CAD build for the part. Positions are in the model's coordinates, mm. A direction names the side the tool comes from. Coordinates: 2 decimals unless noted, no trailing zeros. Order: outer loops, then holes, each group sorted by start corner. A loop starts at its lowest first (then second) coordinate and runs counter-clockwise, first axis right, second up. Notation, with made-up numbers: M 80.5,-39.75 L 131.5,-39.75 A14 cw 131.5,-33.75 Z; hole C 43,62.5 d7. An arc over 180 degrees is marked long. One line per item, written item: value.
from build123d import *

# Parameters (mm, degrees)
F1_DEPTH = 40
F3_DEPTH = 360
F3_TAPER = -3
F4_SIZE  = 10


with BuildPart() as f1:
    # F0 (on Top) → F1 (new body)
    with BuildSketch(Plane.XY):
        with BuildLine():
            Line((348.3026485145, 356.2960825861), (-11.6973514855, 356.2960825861))
            ThreePointArc((-11.6973514855, 356.2960825861), (-25.8394871092, 350.4382182098), (-31.6973514855, 336.2960825861))
            Line((-31.6973514855, 336.2960825861), (-31.6973514855, -23.7039174139))
            ThreePointArc((-31.6973514855, -23.7039174139), (-25.8394871092, -37.8460530377), (-11.6973514855, -43.7039174139))
            Line((-11.6973514855, -43.7039174139), (348.3026485145, -43.7039174139))
            ThreePointArc((348.3026485145, -43.7039174139), (362.4447841382, -37.8460530377), (368.3026485145, -23.7039174139))
            Line((368.3026485145, -23.7039174139), (368.3026485145, 336.2960825861))
            ThreePointArc((368.3026485145, 336.2960825861), (362.4447841382, 350.4382182098), (348.3026485145, 356.2960825861))
        make_face()
    extrude(amount=F1_DEPTH)

    # F2 (on face) → F3 (join)
    with BuildSketch(Plane(origin=(0, 0, 0), x_dir=(1, 0, 0), z_dir=(0, 0, -1))):
        with BuildLine():
            Line((40.8026485145, 3.7039174139), (15.8026485145, 3.7039174139))
            ThreePointArc((15.8026485145, 3.7039174139), (10.4993476556, 1.5072182728), (8.3026485145, -3.7960825861))
            Line((8.3026485145, -3.7960825861), (8.3026485145, -28.7960825861))
            ThreePointArc((8.3026485145, -28.7960825861), (10.4993476556, -34.0993834449), (15.8026485145, -36.2960825861))
            Line((15.8026485145, -36.2960825861), (40.8026485145, -36.2960825861))
            ThreePointArc((40.8026485145, -36.2960825861), (46.1059493734, -34.0993834449), (48.3026485145, -28.7960825861))
            Line((48.3026485145, -28.7960825861), (48.3026485145, -3.7960825861))
            ThreePointArc((48.3026485145, -3.7960825861), (46.1059493734, 1.5072182728), (40.8026485145, 3.7039174139))
        make_face()
        with BuildLine():
            ThreePointArc((288.3026485145, -28.7960825861), (290.4993476556, -34.0993834449), (295.8026485145, -36.2960825861))
            Line((295.8026485145, -36.2960825861), (320.8026485145, -36.2960825861))
            ThreePointArc((320.8026485145, -36.2960825861), (326.1059493734, -34.0993834449), (328.3026485145, -28.7960825861))
            Line((328.3026485145, -28.7960825861), (328.3026485145, -3.7960825861))
            ThreePointArc((328.3026485145, -3.7960825861), (326.1059493734, 1.5072182728), (320.8026485145, 3.7039174139))
            Line((320.8026485145, 3.7039174139), (295.8026485145, 3.7039174139))
            ThreePointArc((295.8026485145, 3.7039174139), (290.4993476556, 1.5072182728), (288.3026485145, -3.7960825861))
            Line((288.3026485145, -3.7960825861), (288.3026485145, -28.7960825861))
        make_face()
        with BuildLine():
            ThreePointArc((288.3026485145, -308.7960825861), (290.4993476556, -314.0993834449), (295.8026485145, -316.2960825861))
            Line((295.8026485145, -316.2960825861), (320.8026485145, -316.2960825861))
            ThreePointArc((320.8026485145, -316.2960825861), (326.1059493734, -314.0993834449), (328.3026485145, -308.7960825861))
            Line((328.3026485145, -308.7960825861), (328.3026485145, -283.7960825861))
            ThreePointArc((328.3026485145, -283.7960825861), (326.1059493734, -278.4927817272), (320.8026485145, -276.2960825861))
            Line((320.8026485145, -276.2960825861), (295.8026485145, -276.2960825861))
            ThreePointArc((295.8026485145, -276.2960825861), (290.4993476556, -278.4927817272), (288.3026485145, -283.7960825861))
            Line((288.3026485145, -283.7960825861), (288.3026485145, -308.7960825861))
        make_face()
        with BuildLine():
            ThreePointArc((8.3026485145, -308.7960825861), (10.4993476556, -314.0993834449), (15.8026485145, -316.2960825861))
            Line((15.8026485145, -316.2960825861), (40.8026485145, -316.2960825861))
            ThreePointArc((40.8026485145, -316.2960825861), (46.1059493734, -314.0993834449), (48.3026485145, -308.7960825861))
            Line((48.3026485145, -308.7960825861), (48.3026485145, -283.7960825861))
            ThreePointArc((48.3026485145, -283.7960825861), (46.1059493734, -278.4927817272), (40.8026485145, -276.2960825861))
            Line((40.8026485145, -276.2960825861), (15.8026485145, -276.2960825861))
            ThreePointArc((15.8026485145, -276.2960825861), (10.4993476556, -278.4927817272), (8.3026485145, -283.7960825861))
            Line((8.3026485145, -283.7960825861), (8.3026485145, -308.7960825861))
        make_face()
    extrude(amount=F3_DEPTH, taper=F3_TAPER)

    # F4
    f4_edges = [f1.edges().sort_by_distance(p)[0] for p in [
        (368.302649, 156.296083, 40),
        (362.444784, 350.438218, 40),
        (168.302649, 356.296083, 40),
        (-25.839487, 350.438218, 40),
        (-31.697351, 156.296083, 40),
        (-25.839487, -37.846053, 40),
        (168.302649, -43.703917, 40),
        (362.444784, -37.846053, 40),
    ]]
    chamfer(f4_edges, length=F4_SIZE)


solid = f1.part
Q1. Which spindle directions (+Z, -Z, +X, -X, +Y, -Y) get a long thin tool onto all of the face, cutting with end or side? Do faces 1 (the face through (28.13, 45.86, -182.52)), 2 (the face through (52.736, 40.995, -182.52)), 3 (the face through (333, -8.14, -182.52)), 4 (the face through (3.604, 40.73, -182.52)), 5 (the face through (-1.263, 296.121, -182.52)). Say none if no direction does.
Recorded:
face 1: +X, -X
face 2: none
face 3: +X, -Y
face 4: -X
face 5: -X, +Y, -Y
Q2. Mould opens along X. For faces 6 (the face through (-25.683, 350.593, 14.79)), 7 (the face through (332.736, 40.995, -182.52)), 8 (the face through (278.737, 16.121, -182.52)) say: released by +X, released by -X, zero draft, split by the parting line, or undercut.
Recorded:
face 6: released by -X
face 7: released by +X
face 8: undercut
Q3. Slice it at A-A (z = -190). Give the number of separate pieces and of enclosed holes in the cut face, plus the area to 3 significant figures.
Recorded:
separate pieces: 4
enclosed holes: 0
area: 13,300 mm^2
Q4. Drill centre lines: line 1 along Z through (x, y) = (114, 319); line 2 along Y through (x, z) = (320.5, -94.5); line 3 along X through (y, z) = (279, -318). Where is each one in solid material? Low to high.
Recorded:
line 1: z = 0 to 40
line 2: y = -8.66 to 41.25, 271.34 to 321.25
line 3: x = -7.88 to 64.49, 272.12 to 344.49
Q5. Slice it at B-B (y = 81.5). List the corners of the cut face in (x, z), plus the area to 3 significant figures.
Recorded:
outline: M -31.7,0 L 368.3,0 L 368.3,30 L 358.3,40 L -21.7,40 L -31.7,30 Z
area: 15,900 mm^2
Q6. Pin check, flat tips, straight feed: pin 1 Ø1.5 at (x, y) = (225, 123.5) entering from -Z; pin 2 Ø3 at (x, z) = (294.5, -19.5) entering from +Y. Stop position of each tip, or through.
Recorded:
pin 1: stops at z = 0
pin 2: stops at y = 317.37
Q7. Slice it at C-C (x = 242). List the corners of the cut face in (y, z).
Recorded:
outline: M -43.7,0 L 356.3,0 L 356.3,30 L 346.3,40 L -33.7,40 L -43.7,30 Z
